Source: CAD feature listing. Evaluate the final solid. Frame: model axes, mm. A direction names the side the tool comes from. Give positions to 0.01 mm unless a question says otherwise; leave off trailing zeros. Loops run counter-clockwise (first coordinate to the right, second up) from the corner with the lowest first, then second, coordinate; pieces in that order, holes last. Notation, with made-up numbers: (-14, -32) -> (37, -32) arc R18 ccw to (37, -9) -> close; hole circle Ø5 at (77, 69). An arc over 180 degrees is marked (long way). Return JSON: item names as keys, results as strings. Group by question number.
```python
from build123d import *

# Parameters (mm, degrees)
F0_R     = 45
F1_DEPTH = 10
F2_R     = 11
F3_DEPTH = 11
F5_D     = 8.2
F7_D     = 5.3
F8_R     = 2.25
F9_DEPTH = 50


# Not quite as in the source:
# - a feature names something its author has since deleted; it is built from what else it names


with BuildPart() as f1:
    # F0 (on Top) → F1 (new body)
    with BuildSketch(Plane.XY):
        Circle(F0_R)
    extrude(amount=F1_DEPTH)

    # F2 (on face) → F3 (join)
    with BuildSketch(Plane.XY.offset(10)):
        Circle(F2_R)
    extrude(amount=F3_DEPTH)

    # F5 (through all)
    with Locations(Plane.XY.offset(21)):
        with Locations((0, 0)):
            Hole(F5_D / 2)

    # F7 (through all)
    with Locations(Plane.XY.offset(10)):
        with Locations((0, 17), (16.167960777, 5.2532889044), (9.992349289, -13.7532889044), (-9.992349289, -13.7532889044), (-16.167960777, 5.2532889044), (35.1890911029, 11.4336287919), (21.7480543348, -29.9336287919), (-21.7480543348, -29.9336287919), (-35.1890911029, 11.4336287919), (0, 37)):
            Hole(F7_D / 2)

    # F8 (on Right) → F9 (cut, symmetric)
    with BuildSketch(Plane.YZ):
        with Locations((0, 17)):
            Circle(F8_R)
    extrude(amount=F9_DEPTH, both=True, mode=Mode.SUBTRACT)


solid = f1.part
```
1) Mould query, pull axis Y, two halves, no side actions, for faces 3 (the face through (9, 1, 0)), 4 (the face through (23.7, -28.14, 4.93)), 5 (the face through (20.765, -39.923, 4.93)), 6 (the face through (-7.889, -15.366, 4.93)). Classes: released by +Y, released by -Y, zero draft, split by the parting line, or undercut.
2) Contact query for flat-ended pins moving along their axis: P1, Ø3, axis at x = -21.75, y = -29.93, coming from the +Z side; P2, Ø10, axis at x = 30.5, z = 3, coming from the -Y side; P3, Ø7, axis at y = 0, z = 17, coming from the +X side; P4, Ø3, axis at y = -31, z = 9, coming from the +X side. Output: stop coordinate, or through.
3) Reachability of faces 1 (the face through (10.161, -4.213, 15.423)), 2 (the face through (-21.403, -27.306, 4.93)) from +Z, -Z, +X, -X, +Y, -Y: full face, straight path, thin tool, end or side. Return the list, or none.
4) Cut plane B-B on y = 0. Return loops of the section in (x, z), then the cut area to 3 significant figures.
5) Cut plane A-A on x = 0. Return loops of the section in (y, z).
6) Cut plane D-D on z = 17. Return loops of the section in (x, y), then the cut area to 3 significant figures.
7) Cut plane C-C on x = -34.5. Return loops of the section in (y, z), then the cut area to 3 significant figures.
8) Material intervals for line 1 (Y direction, x = 0, z = 7.75); line 2 (X direction, y = 5.5, z = 1.75); line 3 (X direction, y = 9.5, z = 6), sorted ascending.
Calculated:
{
 "1": {"face 3": "zero draft", "face 4": "undercut", "face 5": "split by the parting line", "face 6": "undercut"},
 "2": {"P1": "through", "P2": "y = -37.08", "P3": "x = 11", "P4": "x = 33.98"},
 "3": {"face 1": "+Z", "face 2": "+Z, -Z"},
 "4": {"outline": "(-45, 0) -> (-4.1, 0) -> (-4.1, 14.75) -> (-11, 14.75) -> (-11, 10) -> (-45, 10) -> close; (-11, 19.25) -> (-4.1, 19.25) -> (-4.1, 21) -> (-11, 21) -> close; (4.1, 0) -> (45, 0) -> (45, 10) -> (11, 10) -> (11, 14.75) -> (4.1, 14.75) -> close; (4.1, 19.25) -> (11, 19.25) -> (11, 21) -> (4.1, 21) -> close", "area": "908 mm2"},
 "5": {"outline": "(-45, 0) -> (-4.1, 0) -> (-4.1, 21) -> (-11, 21) -> (-11, 10) -> (-45, 10) -> close; (4.1, 0) -> (14.35, 0) -> (14.35, 10) -> (11, 10) -> (11, 21) -> (4.1, 21) -> close; (19.65, 0) -> (34.35, 0) -> (34.35, 10) -> (19.65, 10) -> close; (39.65, 0) -> (45, 0) -> (45, 10) -> (39.65, 10) -> close"},
 "6": {"outline": "(-10.77, -2.25) arc R11 ccw to (10.77, -2.25) -> (3.43, -2.25) arc R4.1 cw to (-3.43, -2.25) -> close; (-10.77, 2.25) -> (-3.43, 2.25) arc R4.1 cw to (3.43, 2.25) -> (10.77, 2.25) arc R11 ccw to start", "area": "264 mm2"},
 "7": {"outline": "(-28.89, 0) -> (8.87, 0) -> (8.87, 10) -> (-28.89, 10) -> close; (13.99, 0) -> (28.89, 0) -> (28.89, 10) -> (13.99, 10) -> close", "area": "527 mm2"},
 "8": {"line 1": "-45 to -4.1, 4.1 to 14.35, 19.65 to 34.35, 39.65 to 45", "line 2": "-44.66 to -18.81, -13.53 to 13.53, 18.81 to 44.66", "line 3": "-43.99 to -37, -33.38 to 33.38, 37 to 43.99"}
}
